Source: CAD feature listing. Evaluate the final solid. Frame: model axes, mm. Face numbers are marked on the shaded views. A direction names the side the tool comes from. Round coordinates to 2 decimals unless told otherwise and drop trailing zeros. Order: outer loops, then holes, each group sorted by start corner. A loop starts at its lowest first (then second) coordinate and runs counter-clockwise, first axis right, second up. Notation, with made-up numbers: (-35, 63.5) - (8, 63.5) arc R18 cw to (8, 80.5) - close; hole circle Ø9 at (42.25, -11). An arc over 180 degrees is marked (long way). Put each result on its own line as item: value. Start each with the question number.
1) Section B-B on y = -45.5. Output: boundary loops of the cut face in (x, z).
2) Mould query, pull axis X, two halves, no side actions, for the marked faces 3, 4, 5 and 6. Classes: +X half, -X half, draft (parallel to the pull), parting line (faces both ways), or undercut.
3) Access query for the marked faces 1 and 2. Directions: +Z, -Z, +X, -X, +Y, -Y. A direction counts if a zero-diameter tool reaches every point of the face in a straight line with its end or side. Return the directions, or none.
4) Section A-A on z = -1. Output: boundary loops of the cut face in (x, y), then the cut area to 3 significant figures.
5) Line query: probe 1 along Z at (x, y) = (21, -10.5); probe 2 along Z at (x, y) = (30.5, -10); probe 3 along Z at (x, y) = (48, -52.5). Output: solid intervals per line, ascending. Write a range as [from, to].
6) Section C-C on x = -37. Output: boundary loops of the cut face in (y, z), then the cut area to 3 significant figures.
7) Contact query for flat-ended pins moving along their axis: P1, Ø8, axis at y = 43.5, z = 7, coming from the +X side; P2, Ø9, axis at y = 6, z = 22.5, coming from the +X side; P3, Ø25, axis at x = 6, z = 28, coming from the +Y side; P4, Ø12, axis at x = 58.5, z = 22.5, coming from the -Y side. Output: stop coordinate, or through.
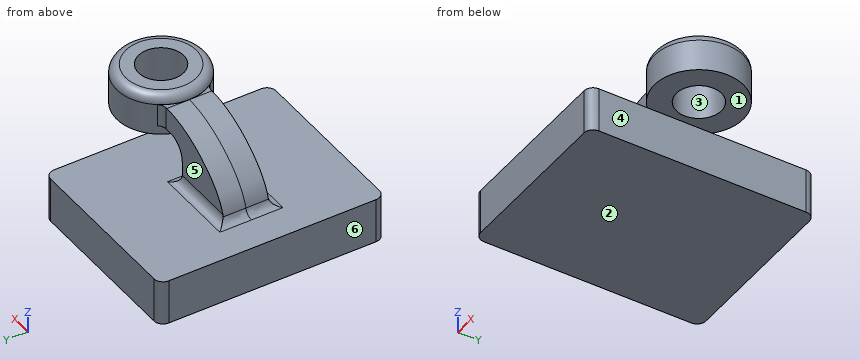
```python
from build123d import *

# Parameters (mm, degrees)
F1_DEPTH  = 63.5
F2_DEPTH  = 63.5
F3_DEPTH  = 12.7
F5_R      = 5.08
F6_R      = 5.08
F7_R      = 5.07999
F10_D     = 25.4
F10_DEPTH = 22.8609980474


# Not quite as in the source:
# - a fillet or chamfer is up to 0.001 mm smaller than in the source, because OpenCascade refuses the exact size


with BuildPart() as f1:
    # F0 (on Front) → F1 (new body, symmetric)
    with BuildSketch(Plane.XZ):
        Polygon((-27.7423580625, 12.7), (-50.8, 12.7), (-50.8, -12.7), (50.8, -12.7), (50.8, 12.7), (9.0188104659, 12.7), align=None)
    extrude(amount=F1_DEPTH, both=True)

    # F0 (on Front) → F2 (join, symmetric)
    with BuildSketch(Plane.XZ):
        Polygon((-27.7423580625, 12.7), (-50.8, 12.7), (-50.8, -12.7), (50.8, -12.7), (50.8, 12.7), (9.0188104659, 12.7), align=None)
    extrude(amount=F2_DEPTH, both=True)

    # F0 (on Front) → F3 (join, symmetric)
    with BuildSketch(Plane.XZ):
        with BuildLine():
            add(Edge.make_bspline(
                [(-27.7423580625, 12.7), (-27.7423580625, 29.5749301373), (-0.0054883666, 49.0460789908), (22.6876754314, 49.0499310609)],
                knots=[0, 0, 0, 0, 62.1644632252, 62.1644632252, 62.1644632252, 62.1644632252], degree=3))
            Line((-27.7423580625, 12.7), (9.0188104659, 12.7))
            Line((9.0188104659, 12.7), (9.0188104659, 26.0071345331))
            ThreePointArc((9.0188104659, 26.0071345331), (12.0481455999, 33.3205964986), (19.3616075654, 36.3499316326))
            Line((19.3616075654, 36.3499316326), (22.6876754314, 36.3499316326))
            Line((22.6876754314, 36.3499316326), (22.6876754314, 49.0499310609))
        make_face()
        with BuildLine():
            add(Edge.make_bspline(
                [(22.6876754314, 49.0499310609), (22.689920498, 49.049931442), (22.6921655153, 49.0499316326), (22.6944104832, 49.0499316326)],
                knots=[62.1644632252, 62.1644632252, 62.1644632252, 62.1644632252, 62.1706132431, 62.1706132431, 62.1706132431, 62.1706132431], degree=3))
            Line((22.6876754314, 49.0499310609), (22.6876754314, 36.3499316326))
            Line((22.6876754314, 36.3499316326), (47.668707557, 36.3499316326))
            Line((47.668707557, 36.3499316326), (47.668707557, 49.0499316326))
            Line((47.668707557, 49.0499316326), (22.6944104832, 49.0499316326))
        make_face()
    extrude(amount=F3_DEPTH, both=True)

    # F0 (on Front) → F4 (revolve)
    with BuildSketch(Plane.XZ):
        Polygon((72.6497396827, 54.1299306562), (47.668707557, 54.1299306562), (47.668707557, 49.0499316326), (47.668707557, 36.3499316326), (47.668707557, 31.2699326089), (72.6497396827, 31.2699326089), align=None)
    revolve(axis=Axis((47.668707557, 0, 42.6999316326), (0, 0, -1)))

    # F5
    f5_edges = [f1.edges().sort_by_distance(p)[0] for p in [
        (-9.361774, -12.7, 12.7),
        (9.01881, 0, 12.7),
        (-27.742358, 6.35, 12.7),
        (-27.742358, -6.35, 12.7),
        (-9.361774, 12.7, 12.7),
        (-50.8, -63.5, 0),
        (-50.8, 63.5, 0),
        (50.8, -63.5, 0),
        (50.8, 63.5, 0),
    ]]
    fillet(f5_edges, radius=F5_R)

    # F6
    f6_edges = [f1.edges().sort_by_distance(p)[0] for p in [
        (26.156805, -12.7, 42.699932),
        (26.156805, 12.7, 42.699932),
    ]]
    fillet(f6_edges, radius=F6_R)

    # F7 (radius 5.08 in the source; OpenCascade refuses exactly that, so slightly less here)
    f7_edges = [f1.edges().sort_by_distance(p)[0] for p in [
        (22.687675, 0, 54.129931),
    ]]
    fillet(f7_edges, radius=F7_R)

    # F10 (through all, one way)
    with BuildSketch(Plane(origin=(0, 0, 31.2699326089), x_dir=(1, 0, 0), z_dir=(0, 0, -1))):
        with Locations((47.61569947, -0.0454496221)):
            Circle(F10_D / 2)
    extrude(amount=-F10_DEPTH, mode=Mode.SUBTRACT)


solid = f1.part
```
Answer sheet:
1. outline: (-50.8, -12.7) - (50.8, -12.7) - (50.8, 12.7) - (-50.8, 12.7) - close
2. face 3: undercut
2. face 4: +X half
2. face 5: draft
2. face 6: -X half
3. face 1: +X, +Y, -Y
3. face 2: -Z, +X, -X, +Y, -Y
4. outline: (-50.8, -58.42) arc R5.08 ccw to (-45.72, -63.5) - (45.72, -63.5) arc R5.08 ccw to (50.8, -58.42) - (50.8, 58.42) arc R5.08 ccw to (45.72, 63.5) - (-45.72, 63.5) arc R5.08 ccw to (-50.8, 58.42) - close
4. area: 12,900 mm^2
5. probe 1: [-12.7, 12.7], [36.35, 49.01]
5. probe 2: [-12.7, 12.7], [31.27, 54.13]
5. probe 3: [-12.7, 12.7]
6. outline: (-63.5, -12.7) - (63.5, -12.7) - (63.5, 12.7) - (-63.5, 12.7) - close
6. area: 3,230 mm^2
7. P1: x = 50.8
7. P2: x = 9.07
7. P3: y = 13.24
7. P4: through
